The model under review builds one solid part; all positions refer to its coordinate system, in mm. Coordinates: 2 decimals unless noted, no trailing zeros. Loops run counter-clockwise (first coordinate to the right, second up) from the corner with the lowest first, then second, coordinate; pieces in that order, holes last. Notation, with made-up numbers: M -12,81.25 L -3,81.25 A8 ccw -3,96.25 Z; hole C 83.5,67 d2. An arc over 180 degrees is marked long. Return JSON: item names as keys, results as strings.
```python
from build123d import *

# Parameters (mm, degrees)
SKETCH1_R               = 45
SKETCH1_R_2             = 42
BOSS_EXTRUDE1_DEPTH     = 170
CUT_EXTRUDE1_DEPTH      = 182.521348607
CUT_EXTRUDE1_DEPTH_BACK = 182.521348607
SKETCH2_R               = 2
SKETCH2_R_2             = 1.5


with BuildPart() as part:
    # Sketch1 → Boss-Extrude1 (new body)
    with BuildSketch(Plane(origin=(0, 0, 0), x_dir=(1, 0, 0), z_dir=(0, 1, 0))):
        with Locations(Location((0, 0, 0), (0, 0, 270))):
            Circle(SKETCH1_R)
        with Locations(Location((0, 0, 0), (0, 0, 270))):
            Circle(SKETCH1_R_2, mode=Mode.SUBTRACT)
    extrude(amount=-BOSS_EXTRUDE1_DEPTH)

    # Sketch2 → Cut-Extrude1 (cut, two sides: drawn at the far end of the back side and taken through both)
    with BuildSketch(Plane.XY.offset(-CUT_EXTRUDE1_DEPTH_BACK)):
        with Locations((0, -164)):
            Circle(SKETCH2_R)
        with Locations((-20, -15)):
            Circle(SKETCH2_R_2)
        with Locations((20, -15)):
            Circle(SKETCH2_R_2)
    extrude(amount=CUT_EXTRUDE1_DEPTH + CUT_EXTRUDE1_DEPTH_BACK, mode=Mode.SUBTRACT)


solid = part.part
```
1. The part is to be moulded in two halves that separate along Y. For faces 1 (the face through (-40, -170, -14)), 2 (the face through (-40, 0, -14)), 3 (the face through (0.923, -165.774, 43.455)), say which applies: released by +Y, released by -Y, zero draft, split by the parting line, or undercut.
Check values:
{"face 1": "released by -Y", "face 2": "released by +Y", "face 3": "undercut"}
2. To check wall thickness, follow line 1 (Z direction, x = 0, y = -88); line 2 (Y direction, x = -20, z = 39.65); line 3 (Z direction, x = -14, y = -57). State the ranges of each line that lie inside material, in increasing order.
Check values:
{"line 1": "-45 to -42, 42 to 45", "line 2": "-170 to -16.5, -13.5 to 0", "line 3": "-42.77 to -39.6, 39.6 to 42.77"}
3. Add section A-A on x = 0. Give the boundary of the cut face in (y, z), plus the area to 3 significant figures.
Check values:
{"outline": "M -170,-45 L -166,-45 L -166,-42 L -170,-42 Z; M -170,42 L -166,42 L -166,45 L -170,45 Z; M -162,-45 L 0,-45 L 0,-42 L -162,-42 Z; M -162,42 L 0,42 L 0,45 L -162,45 Z", "area": "996 mm²"}
4. Add section B-B on z = 0. Give the boundary of the cut face in (x, y).
Check values:
{"outline": "M -45,-170 L -42,-170 L -42,0 L -45,0 Z; M 42,-170 L 45,-170 L 45,0 L 42,0 Z"}
5. Add section D-D on y = -63.5. Give the boundary of the cut face in (x, z), plus the area to 3 significant figures.
Check values:
{"outline": "C 0,0 d90; hole C 0,0 d84", "area": "820 mm²"}
6. Insertion check: pin 1 Ø12 at (x, y) = (-31.5, -36.5) entering from +Z; pin 2 Ø8 at (x, z) = (-31.5, -34) entering from +Y; pin 3 Ø1 at (x, y) = (26.5, -122) entering from -Z; pin 4 Ø4 at (x, y) = (29.5, -60.5) entering from +Z. Each pin has a flat end and moves straight along its axis. Give the tip position at first contact, or say it passes through.
Check values:
{"pin 1": "z = 37.08", "pin 2": "y = 0", "pin 3": "z = -36.73", "pin 4": "z = 35.62"}
